The figure shows three views and two pictorial views of one solid part (mm, origin at its lowest corner). Answer the questions. A direction names the side the tool comes from. Round coordinates to 2 decimals unless told otherwise and drop trailing zeros. Write each loop counter-clockwise with the first axis right and the second up, starting at its lowest first coordinate (ties: lowest second). Pieces come first, ordered by that corner, then holes.
Item 1: Each of these flat-tipped pins is pushed along its axis until it touches: pin 1 (1.5 mm diameter, centred on x = 81, y = 14, fed in from -Z); pin 2 (1.5 mm diameter, centred on x = 103.5, z = 12, fed in from -Y). Where does it stop, or does it pass through?
Item 2: A tool of negligible diameter and unlimited length cuts with its end or side. For the marked faces 5, 6 and 7, from which of +Z, -Z, +X, -X, +Y, -Y can it reach the whole face along a straight path? Write none if from no direction.
Item 3: Find section C-C on y = 44. Give the vertices of the cut face in (x, z).
Item 4: For a pull along X with two mould halves and no side action, classify the marked faces 1, 2, 3 and 4 as +X half, -X half, draft (parallel to the pull), parting line (faces both ways), or undercut.
Item 5: Find the intervals of material crossed by probe 1 along X at (y, z) = (57, 23.5); probe 2 along X at (y, z) = (22, 29); probe 3 along Z at (x, y) = (126, 28.5), in increasing order.
Item 6: Find section A-A on y = 6. Give the vertices of the cut face in (x, z) (1 decimal), then the cut area to 3 significant figures.
Item 7: Find section D-D on y = 53.5. Give the vertices of the cut face in (x, z).
Item 8: Find section B-B on z = 48. Give the vertices of the cut face in (x, y).
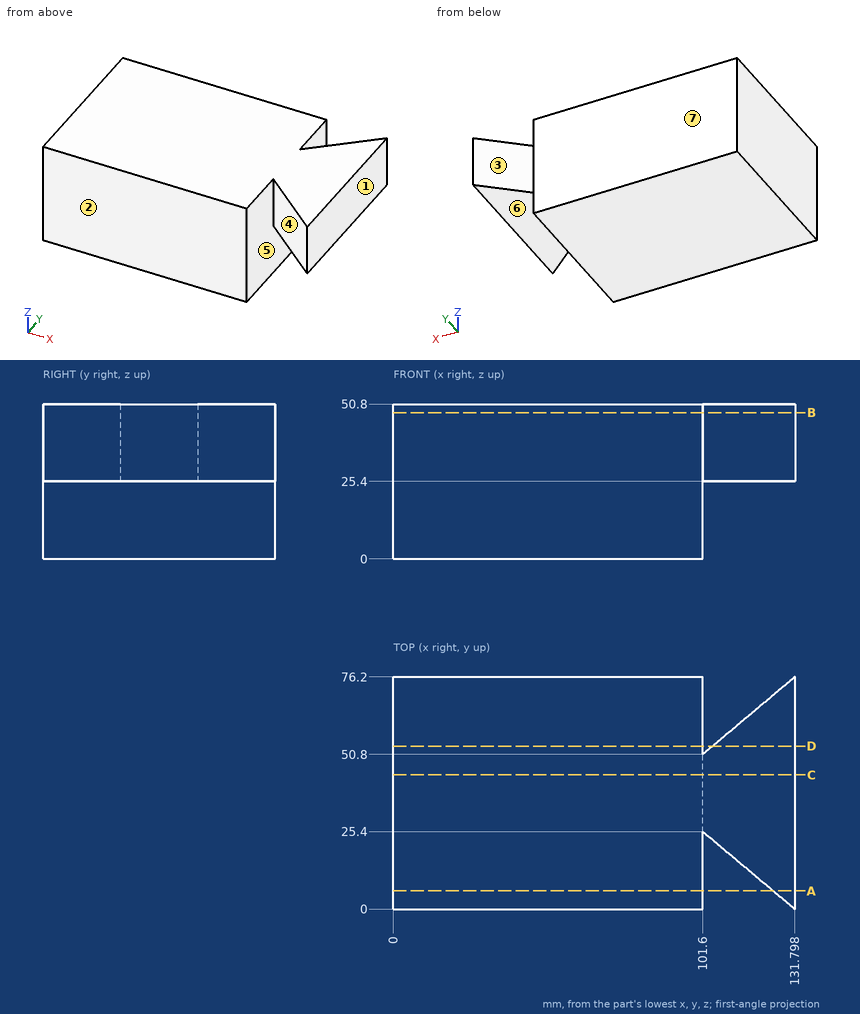
Check values:
1. pin 1: stops at z = 0
1. pin 2: passes through
2. face 5: -Z
2. face 6: -Z, +X, +Y, -Y
2. face 7: +Z, -Z, +X, -X, +Y
3. outline: (0, 0) - (101.6, 0) - (101.6, 25.4) - (131.8, 25.4) - (131.8, 50.8) - (0, 50.8) - close
4. face 1: +X half
4. face 2: draft
4. face 3: undercut
4. face 4: undercut
5. probe 1: x = 0 to 101.6
5. probe 2: x = 0 to 101.6, 105.64 to 131.8
5. probe 3: z = 25.4 to 50.8
6. outline: (0, 0) - (101.6, 0) - (101.6, 50.8) - (0, 50.8) - close; (124.7, 25.4) - (131.8, 25.4) - (131.8, 50.8) - (124.7, 50.8) - close
6. area: 5,340 mm2
7. outline: (0, 0) - (101.6, 0) - (101.6, 50.8) - (0, 50.8) - close; (104.81, 25.4) - (131.8, 25.4) - (131.8, 50.8) - (104.81, 50.8) - close
8. outline: (0, 0) - (101.6, 0) - (101.6, 25.4) - (131.8, 0) - (131.8, 76.2) - (101.6, 50.8) - (101.6, 76.2) - (0, 76.2) - close
